The model under review builds one solid part; all positions refer to its coordinate system, in mm. A direction names the side the tool comes from. Give positions to 0.01 mm unless a question says otherwise; leave off trailing zeros. Order: outer loops, then holes, each group sorted by start corner. A loop starts at its lowest first (then second) coordinate and runs counter-clockwise, first axis right, second up. Notation, with made-up numbers: (-17, 17.5) - (16, 17.5) arc R19 ccw to (16, 23.5) - close; hole circle Ø4 at (56.25, -15.75). An arc over 180 degrees is marked (long way). Answer as CSV lines item,"result". Start each with the question number.
from build123d import *

# Parameters (mm, degrees)
SKETCH1_W           = 39.8
SKETCH1_H           = 39.8
BOSS_EXTRUDE1_DEPTH = 4
FILLET1_R           = 6
SKETCH2_R           = 2
BOSS_EXTRUDE2_DEPTH = 18


with BuildPart() as part:
    # Sketch1 → Boss-Extrude1 (new body)
    with BuildSketch(Plane(origin=(0, 0, 0), x_dir=(1, 0, 0), z_dir=(0, 1, 0))):
        Rectangle(SKETCH1_W, SKETCH1_H)
    extrude(amount=BOSS_EXTRUDE1_DEPTH)

    # Fillet1
    fillet1_edges = [part.edges().sort_by_distance(p)[0] for p in [
        (19.9, 2, 19.9),
        (-19.9, 2, 19.9),
        (-19.9, 2, -19.9),
        (19.9, 2, -19.9),
    ]]
    fillet(fillet1_edges, radius=FILLET1_R)

    # Sketch2 → Boss-Extrude2 (add)
    with BuildSketch(Plane(origin=(0, 4, 0), x_dir=(1, 0, 0), z_dir=(0, 1, 0))):
        with Locations((-10, 10)):
            Circle(SKETCH2_R)
        with Locations((10, 10)):
            Circle(SKETCH2_R)
        with Locations((10, -10)):
            Circle(SKETCH2_R)
        with Locations((-10, -10)):
            Circle(SKETCH2_R)
    extrude(amount=BOSS_EXTRUDE2_DEPTH)


solid = part.part
Item 1: Mouldability with a two-part tool opening along Z and no side actions: class faces 1 (the face through (0, 0, 0)), 2 (the face through (0, 2, 19.9)), 3 (the face through (10, 13, -12)) as released by +Z, released by -Z, zero draft, split by the parting line, or undercut.
Item 2: Take a section at D-D on y = 6. Write out the cut boundary in (x, z).
Item 3: Machinability: for faces 4 (the face through (0, 4, 0)), 5 (the face through (10, 22, -10)), which of the approach directions +Z, -Z, +X, -X, +Y, -Y give a long, thin tool a straight path to every point of the face, cutting with its end or side? Answer none if there is none.
Item 4: Take a section at B-B on y = 3.25. Write out the cut boundary in (x, z), and give its area (3 significant figures).
Item 5: Take a section at A-A on z = -10. Write out the cut boundary in (x, y).
Item 6: For line 1 along X through (y, z) = (8.5, -10); line 2 along Y through (x, z) = (-10, 6); line 3 along Z through (x, y) = (-11.5, 6), list the stretches that pass through material, from the lowest coordinate up.
Item 7: Clearance check with flat-ended pins moving along their axes: pin 1 (10 mm diameter, centred on y = 14, z = -2.5, fed in from -X); pin 2 (6 mm diameter, centred on x = 7.5, y = 17.5, fed in from +Z); pin 3 (5 mm diameter, centred on y = 8, z = 6, fed in from +X). State where each tip first meets the part, or that it passes through.
Item 8: Take a section at C-C on x = 10. Write out the cut boundary in (y, z), and give its area (3 significant figures).
Data:
1,face 1,"zero draft"
1,face 2,"released by +Z"
1,face 3,"undercut"
2,outline,"circle Ø4 at (-10, -10); circle Ø4 at (-10, 10); circle Ø4 at (10, -10); circle Ø4 at (10, 10)"
3,face 4,"+Y"
3,face 5,"+Z, -Z, +X, -X, +Y"
4,outline,"(-19.9, -13.9) arc R6 ccw to (-13.9, -19.9) - (13.9, -19.9) arc R6 ccw to (19.9, -13.9) - (19.9, 13.9) arc R6 ccw to (13.9, 19.9) - (-13.9, 19.9) arc R6 ccw to (-19.9, 13.9) - close"
4,area,"1,550 mm^2"
5,outline,"(-19.9, 0) - (19.9, 0) - (19.9, 4) - (12, 4) - (12, 22) - (8, 22) - (8, 4) - (-8, 4) - (-8, 22) - (-12, 22) - (-12, 4) - (-19.9, 4) - close"
6,line 1,"x = -12 to -8, 8 to 12"
6,line 2,"y = 0 to 4"
6,line 3,"z = -11.32 to -8.68, 8.68 to 11.32"
7,pin 1,"passes through"
7,pin 2,"stops at z = 12"
7,pin 3,"stops at x = 11.32"
8,outline,"(0, -19.9) - (4, -19.9) - (4, -12) - (22, -12) - (22, -8) - (4, -8) - (4, 8) - (22, 8) - (22, 12) - (4, 12) - (4, 19.9) - (0, 19.9) - close"
8,area,"303 mm^2"
